The listing builds one solid part. Answer for the finished solid, in the listing's coordinates (mm). Coordinates: 2 decimals unless noted, no trailing zeros. Order: outer loops, then holes, each group sorted by start corner. A loop starts at its lowest first (then second) coordinate and runs counter-clockwise, first axis right, second up. Notation, with made-up numbers: (-1, 1.5) -> (51, 1.5) arc R17 cw to (51, 20.5) -> close; hole circle Ø6 at (84, 82.25). An arc over 180 degrees is marked (long way). Write item = value, one per line. Start each with the question number.
Autodesk Inventor part; units mm, degrees
ref_plane "YZ Plane" through (0, 0, 0) normal (1, 0, 0) x (0, 1, 0)
ref_plane "XZ Plane" through (0, 0, 0) normal (0, 1, 0) x (-1, 0, 0)
ref_plane "XY Plane" through (0, 0, 0) normal (0, 0, 1) x (1, 0, 0)
sketch "Sketch1" plane through (0, 0, 0) normal (0, 1, 0) x (-1, 0, 0)
  circle A0 centre (0, 0) radius 31
  circle A1 centre (0, 0) radius 33.5
  dimension "d0" = 62
  dimension "d1" = 67
extrude "Extrusion1" add sketch "Sketch1" along normal blind 23
sketch "Sketch3" plane through (0, 23, 0) normal (0, 1, 0) x (1, 0, 0)
  circle A0 centre (0, 0) radius 31
hole "Hole1" at (0, 23, 0) direction (0, -1, 0) diameter 62 end through all
sketch "Sketch4" plane through (0, 23, 0) normal (0, 1, 0) x (1, 0, 0)
  circle A0 centre (0, 0) radius 9.4443
hole "Hole2" at (0, 23, 0) direction (0, -1, 0) diameter 62 end through all
properties part number "rueda de rolinera"
Item 1: Each of these flat-tipped pins is pushed along its axis until it touches: pin 1 (3 mm diameter, centred on x = -24.5, y = 6, fed in from -Z); pin 2 (4 mm diameter, centred on y = 7.5, z = -8, fed in from -X); pin 3 (6 mm diameter, centred on y = 11, z = 4.5, fed in from +X). Where does it stop, or does it pass through?
Item 2: For a pull along Z with two mould halves and no side action, classify faces 1 (the cylindrical face through (7.262, 11.339, 32.703)), 2 (the cylindrical face through (4.036, 11.339, -30.736)), 3 (the flat face through (-10, 23, -30)) as pulls with the +Z half, pulls with the -Z half, needs draft (parallel to the pull), parting line crosses it, or undercut.
Item 3: Consider probe 1 along Z at (x, y) = (0, 6); probe 2 along Z at (x, y) = (16, 2.5); probe 3 along X at (y, z) = (3.5, 25.5). Determine where each line is inside the solid, lowest interval first.
Item 4: Section C-C, the plane y = 12.5 is taken. Give the vertices of the cut face in (x, z).
Item 5: Section B-B, the plane x = 0 is taken. Give the vertices of the cut face in (y, z).
Item 6: Section A-A, the plane z = 0 is taken. Give the vertices of the cut face in (x, y).
A:
q1.pin_1 = -24.36
q1.pin_2 = -32.96
q1.pin_3 = 33.47
q2.face_1 = parting line crosses it
q2.face_2 = undercut
q2.face_3 = needs draft
q3.probe_1 = -33.5 to -31, 31 to 33.5
q3.probe_2 = -29.43 to -26.55, 26.55 to 29.43
q3.probe_3 = -21.73 to -17.63, 17.63 to 21.73
q4.outline = circle Ø67 at (0, 0); hole circle Ø62 at (0, 0)
q5.outline = (0, -33.5) -> (23, -33.5) -> (23, -31) -> (0, -31) -> close; (0, 31) -> (23, 31) -> (23, 33.5) -> (0, 33.5) -> close
q6.outline = (-33.5, 0) -> (-31, 0) -> (-31, 23) -> (-33.5, 23) -> close; (31, 0) -> (33.5, 0) -> (33.5, 23) -> (31, 23) -> close
